Input: part model. Units: mm. Frame: model coordinates. Face numbers are marked on the shaded views. Coordinates: 2 decimals unless noted, no trailing zeros. Write each loop counter-clockwise with the first axis right and the second up, starting at its lowest first coordinate (ties: lowest second). Pieces come first, ordered by that corner, then holes.
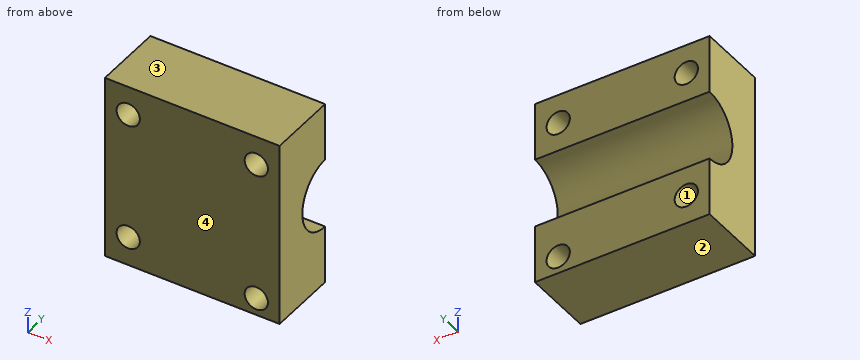
from build123d import *

# Parameters (mm, degrees)
BOSS_EXTRUDE1_DEPTH = 30
SKETCH2_R           = 2
CUT_EXTRUDE1_DEPTH  = 13


with BuildPart() as part:
    # Sketch1 → Boss-Extrude1 (new body)
    with BuildSketch(Plane(origin=(0, 0, 0), x_dir=(0, 0, -1), z_dir=(1, 0, 0))):
        with BuildLine():
            Line((0, 0), (0, 12))
            Line((0, 12), (10, 12))
            ThreePointArc((10, 12), (16, 6), (22, 12))
            Line((22, 12), (32, 12))
            Line((32, 12), (32, 0))
            Line((32, 0), (0, 0))
        make_face()
    extrude(amount=BOSS_EXTRUDE1_DEPTH)

    # Sketch2 → Cut-Extrude1 (cut, through all)
    with BuildSketch(Plane(origin=(0, 12, 0), x_dir=(1, 0, 0), z_dir=(0, 1, 0))):
        with Locations((4, 27)):
            Circle(SKETCH2_R)
        with Locations((26, 29)):
            Circle(SKETCH2_R)
        with Locations((4, 5)):
            Circle(SKETCH2_R)
        with Locations((26, 5)):
            Circle(SKETCH2_R)
    extrude(amount=-CUT_EXTRUDE1_DEPTH, mode=Mode.SUBTRACT)


solid = part.part
Item 1: Section query C-C, the plane y = 8. Return loops of the section in (x, z).
Item 2: Pull-direction query (Z, two-part tool) for the marked faces 1, 2, 3 and 4; classes: released by +Z, released by -Z, zero draft, split by the parting line, or undercut.
Item 3: Section query D-D, the plane y = 2.25. Return loops of the section in (x, z).
Item 4: Section query A-A, the plane x = 26. Return loops of the section in (y, z).
Item 5: Section query B-B, the plane z = -5. Return loops of the section in (x, y), then the cut area to 3 significant figures.
Item 6: Material intervals for line 1 (Z direction, x = 4, y = 2.5); line 2 (X direction, y = 3.75, z = -5); line 3 (Z direction, x = 26, y = 3), sorted ascending.
The answers:
1. outline: (0, -32) - (30, -32) - (30, -20.47) - (0, -20.47) - close; (0, -11.53) - (30, -11.53) - (30, 0) - (0, 0) - close; hole circle Ø4 at (4, -27); hole circle Ø4 at (4, -5); hole circle Ø4 at (26, -29); hole circle Ø4 at (26, -5)
2. face 1: undercut
2. face 2: released by -Z
2. face 3: released by +Z
2. face 4: zero draft
3. outline: (0, -32) - (30, -32) - (30, 0) - (0, 0) - close; hole circle Ø4 at (4, -27); hole circle Ø4 at (4, -5); hole circle Ø4 at (26, -29); hole circle Ø4 at (26, -5)
4. outline: (0, -32) - (12, -32) - (12, -31) - (0, -31) - close; (0, -27) - (12, -27) - (12, -22) arc R6 cw to (12, -10) - (12, -7) - (0, -7) - close; (0, -3) - (12, -3) - (12, 0) - (0, 0) - close
5. outline: (0, 0) - (2, 0) - (2, 12) - (0, 12) - close; (6, 0) - (24, 0) - (24, 12) - (6, 12) - close; (28, 0) - (30, 0) - (30, 12) - (28, 12) - close
5. area: 264 mm2
6. line 1: z = -32 to -29, -25 to -7, -3 to 0
6. line 2: x = 0 to 2, 6 to 24, 28 to 30
6. line 3: z = -32 to -31, -27 to -7, -3 to 0
